Design review of the part built by this model. Coordinates are the model's own, in mm. Face numbers are marked on the shaded views. A direction names the side the tool comes from. Give positions to 0.01 mm unless a question says otherwise; leave off trailing zeros. Order: outer loops, then holes, each group sorted by start corner. A loop starts at its lowest first (then second) coordinate and runs counter-clockwise, first axis right, second up. Notation, with made-up numbers: (43, 1) - (90, 1) arc R33 cw to (90, 37) - close; hole circle Ø9 at (62, 40.25). An arc over 180 degrees is marked (long way). Write each question's results on one line, items separated by ' | '. Start each with the question number.
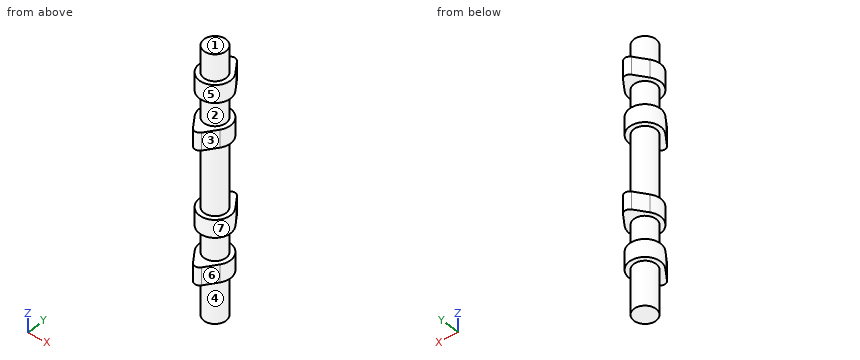
```python
from build123d import *

# Parameters (mm, degrees)
SKETCH1_R           = 6.25
BOSS_EXTRUDE1_DEPTH = 150
SKETCH2_R           = 6.25
BOSS_EXTRUDE2_DEPTH = 10
SKETCH3_R           = 6.25
BOSS_EXTRUDE3_DEPTH = 10
BOSS_EXTRUDE4_DEPTH = 10
BOSS_EXTRUDE5_DEPTH = 10


with BuildPart() as part:
    # Sketch1 → Boss-Extrude1 (new body)
    with BuildSketch(Plane.XY):
        Circle(SKETCH1_R)
    extrude(amount=BOSS_EXTRUDE1_DEPTH)

    # Sketch2 → Boss-Extrude2 (add)
    with BuildSketch(Plane.XY.offset(135)):
        with BuildLine():
            Line((-2.443849423, 11.74), (-7.168624973, 5.104))
            ThreePointArc((-7.168624973, 5.104), (0, -8.8), (7.168624973, 5.104))
            Line((7.168624973, 5.104), (2.443849423, 11.74))
            ThreePointArc((2.443849423, 11.74), (0, 13), (-2.443849423, 11.74))
        make_face()
        Circle(SKETCH2_R, mode=Mode.SUBTRACT)
    extrude(amount=-BOSS_EXTRUDE2_DEPTH)

    # Sketch3 → Boss-Extrude3 (add)
    with BuildSketch(Plane(origin=(0, 0, 110), x_dir=(-1, 0, 0), z_dir=(0, 0, -1))):
        with BuildLine():
            Line((2.443849423, -11.74), (7.168624973, -5.104))
            ThreePointArc((7.168624973, -5.104), (0, 8.8), (-7.168624973, -5.104))
            Line((-7.168624973, -5.104), (-2.443849423, -11.74))
            ThreePointArc((-2.443849423, -11.74), (0, -13), (2.443849423, -11.74))
        make_face()
        Circle(SKETCH3_R, mode=Mode.SUBTRACT)
    extrude(amount=BOSS_EXTRUDE3_DEPTH)

    # Sketch4 → Boss-Extrude4 (add)
    with BuildSketch(Plane(origin=(0, 0, 60), x_dir=(-1, 0, 0), z_dir=(0, 0, -1))):
        with BuildLine():
            Line((-2.443849423, 11.74), (-7.168624973, 5.104))
            ThreePointArc((-7.168624973, 5.104), (0, -8.8), (7.168624973, 5.104))
            Line((7.168624973, 5.104), (2.443849423, 11.74))
            ThreePointArc((2.443849423, 11.74), (0, 13), (-2.443849423, 11.74))
        make_face()
    extrude(amount=BOSS_EXTRUDE4_DEPTH)

    # Sketch5 → Boss-Extrude5 (add)
    with BuildSketch(Plane(origin=(0, 0, 35), x_dir=(-1, 0, 0), z_dir=(0, 0, -1))):
        with BuildLine():
            Line((2.443849423, -11.74), (7.168624973, -5.104))
            ThreePointArc((7.168624973, -5.104), (0, 8.8), (-7.168624973, -5.104))
            Line((-7.168624973, -5.104), (-2.443849423, -11.74))
            ThreePointArc((-2.443849423, -11.74), (0, -13), (2.443849423, -11.74))
        make_face()
    extrude(amount=BOSS_EXTRUDE5_DEPTH)


solid = part.part
```
Q1. Insertion check: pin 1 Ø2 at (y, z) = (7, 101.5) entering from +X; pin 2 Ø4 at (x, y) = (4, 7.5) entering from +Z; pin 3 Ø2 at (x, y) = (6.5, 6) entering from -Z. Each pin has a flat end and moves straight along its axis. Give the tip position at first contact, or say it passes through.
Q2. Machinability: for the marked faces 4, 5, 6 and 7, which of the approach directions +Z, -Z, +X, -X, +Y, -Y give a long, thin tool a straight path to every point of the face, cutting with its end or side? Answer none if there is none.
Q3. Add section C-C (z = 52). Give the boundary of the cut face in (x, y), plus the area to 3 significant figures.
Q4. Draft analysis for pull direction Z (two halves, no side actions). For the marked faces 1, 2 and 3, state which applies: pulls with the +Z half, pulls with the -Z half, needs draft (parallel to the pull), parting line crosses it, or undercut.
Q5. Add section A-A (y = -10.25). Give the boundary of the cut face in (x, z), plus the area to 3 significant figures.
Q6. For line 1 (Z direction, x = 0, y = 8.5); line 2 (Y direction, x = -0.25, z = 106.5); line 3 (Z direction, x = 1, y = 11.75), list the stretches that pass through material, from the lowest coordinate up. Write a range as [from, to].
Q7. Add section B-B (z = 81.5). Give the boundary of the cut face in (x, y), plus the area to 3 significant figures.
Verdict:
1) pin 1: stops at x = 6.44 | pin 2: stops at z = 135 | pin 3: stops at z = 25
2) face 4: -Z | face 5: +Z | face 6: +Z, -Z, +X, -Y | face 7: none
3) outline: (-7.17, 5.1) arc R8.8 ccw (long way) to (7.17, 5.1) - (2.44, 11.74) arc R3 ccw to (-2.44, 11.74) - close | area: 274 mm2
4) face 1: pulls with the +Z half | face 2: undercut | face 3: needs draft
5) outline: (-3.5, 25) - (3.5, 25) - (3.5, 35) - (-3.5, 35) - close; (-3.5, 100) - (3.5, 100) - (3.5, 110) - (-3.5, 110) - close | area: 140 mm2
6) line 1: z = [25, 35], [50, 60], [100, 110], [125, 135] | line 2: y = [-12.99, 8.8] | line 3: z = [50, 60], [125, 135]
7) outline: circle Ø12.5 at (0, 0) | area: 123 mm2
